```python
from build123d import *

# Parameters (mm, degrees)
F0_W     = 14
F0_H     = 16
F1_DEPTH = 1.5
F2_W     = 10.9
F2_H     = 1.4
F3_DEPTH = 15
F5_DEPTH = 25
F6_W     = 4.033105
F6_H     = 2.050732
F6_W_2   = 3.937547
F6_H_2   = 2.08491
F7_DEPTH = 25


with BuildPart() as f1:
    # F0 (on Top) → F1 (new body)
    with BuildSketch(Plane.XY):
        Rectangle(F0_W, F0_H)
    extrude(amount=F1_DEPTH)

    # F2 (on face) → F3 (cut)
    with BuildSketch(Plane.XZ.offset(8)):
        with Locations((-1.45, 0.7)):
            Rectangle(F2_W, F2_H)
    extrude(amount=-F3_DEPTH, mode=Mode.SUBTRACT)

    # F4 (on face) → F5 (cut)
    with BuildSketch(Plane.XY.offset(1.5)):
        Polygon((-7, -8), (4.272356, -8), (4.272356, -7.365542), (3.178632, -7.365542), (2.495055, -6.476892), (-5.947122, -6.476892), (-6.323089, -6.955396), (-7, -6.955396), align=None)
    extrude(amount=-F5_DEPTH, mode=Mode.SUBTRACT)

    # F6 (on face) → F7 (cut)
    with BuildSketch(Plane.XY.offset(1.5)):
        with Locations((-4.313515, -3.946002)):
            Rectangle(F6_W, F6_H)
        with Locations((0.526281, -3.963091)):
            Rectangle(F6_W_2, F6_H_2)
    extrude(amount=-F7_DEPTH, mode=Mode.SUBTRACT)


solid = f1.part
```
Verification items for the finished model (mm, model axes). A direction names the side the tool comes from. Give positions to 0.01 mm unless a question says otherwise; leave off trailing zeros. Write each loop counter-clockwise with the first axis right and the second up, starting at its lowest first coordinate (ties: lowest second). Pieces come first, ordered by that corner, then holes. Notation, with made-up numbers: (66.25, 18.25) - (71.25, 18.25) arc R17 cw to (71.25, 49.25) - close; hole circle Ø7 at (46, -9). An arc over 180 degrees is marked (long way). Put each result on its own line as item: value.
Q1. Section check D-D on x = -2.75. Record the cut outline in (y, z).
Result:
outline: (-6.48, 1.4) - (-4.97, 1.4) - (-4.97, 1.5) - (-6.48, 1.5) - close; (-2.92, 1.4) - (7, 1.4) - (7, 0) - (8, 0) - (8, 1.5) - (-2.92, 1.5) - close
Q2. Scan lines: probe 1 along X at (y, z) = (-7, 0.35); probe 2 along Y at (x, z) = (0.75, 0.1). Record each from-to range of solid material in increasing order. Write a range as from..to.
Result:
probe 1: 4..7
probe 2: 7..8
Q3. Depth check by flat-ended pin: P1, Ø0.5, axis at x = -6.5, z = 0.5, coming from the -Y side. Enter the tip coordinate at first touch or a pass-through.
Result:
P1: y = 7
Q4. Mould release check, pull along X, two halves, no side actions. Record for faces 1 (the face through (7, 0, 1)), 2 (the face through (-2, 7, 1)), 3 (the face through (6, -8, 1)): released by +X, released by -X, zero draft, split by the parting line, or undercut.
Result:
face 1: released by +X
face 2: undercut
face 3: zero draft
Q5. Section check C-C on z = 1.1. Record the cut outline in (x, y), and give its area (3 significant figures).
Result:
outline: (-7, -6.96) - (-6.9, -6.96) - (-6.9, 7) - (4, 7) - (4, -7.37) - (4.27, -7.37) - (4.27, -8) - (7, -8) - (7, 8) - (-7, 8) - close
area: 60.2 mm2
Q6. Section check B-B on y = -3.75. Record the cut outline in (x, z), and give its area (3 significant figures).
Result:
outline: (-7, 0) - (-6.9, 0) - (-6.9, 1.4) - (-6.33, 1.4) - (-6.33, 1.5) - (-7, 1.5) - close; (-2.3, 1.4) - (-1.44, 1.4) - (-1.44, 1.5) - (-2.3, 1.5) - close; (2.5, 1.4) - (4, 1.4) - (4, 0) - (7, 0) - (7, 1.5) - (2.5, 1.5) - close
area: 4.94 mm2
Q7. Set-up check for faces 4 (the face through (4, 0, 1)), 5 (the face through (5, 1, 0)): record each of +Z, -Z, +X, -X, +Y, -Y from which the full face is reachable in a straight line by a thin tool's end or side.
Result:
face 4: -Z, -Y
face 5: -Z, +X, -X, +Y, -Y
Q8. Section check A-A on x = -0.5. Record the cut outline in (y, z).
Result:
outline: (-6.48, 1.4) - (-5.01, 1.4) - (-5.01, 1.5) - (-6.48, 1.5) - close; (-2.92, 1.4) - (7, 1.4) - (7, 0) - (8, 0) - (8, 1.5) - (-2.92, 1.5) - close
